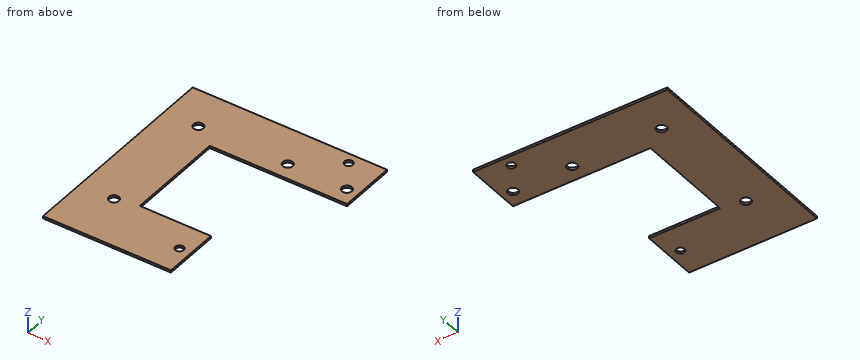
```python
from build123d import *

# Parameters (mm, degrees)
BASE_FLANGE1_DEPTH = 1
SKETCH3_R          = 2.1
SKETCH3_R_2        = 1.75
CUT_EXTRUDE1_DEPTH = 40
SKETCH4_R          = 1.75
CUT_EXTRUDE2_DEPTH = 10


# Sheet-metal steps are written as plain solids
with BuildPart() as part:
    # Sketch1 → Base-Flange1 (new body)
    with BuildSketch(Plane.XY):
        Polygon((0, 24), (-59, 24), (-59, -66), (-35, -66), (-5, -66), (-5, -42), (-35, -42), (-35, 0), (23, 0), (23, 24), align=None)
    extrude(amount=-BASE_FLANGE1_DEPTH)

    # Sketch3 → Cut-Extrude1 (cut)
    with BuildSketch(Plane.XY):
        with Locations((-44.600589414, -43.844308668)):
            Circle(SKETCH3_R)
        with Locations((-44.600589414, 6.892572586)):
            Circle(SKETCH3_R)
        with Locations((-6.896760866, 6.942572586)):
            Circle(SKETCH3_R)
        with Locations((18.060540453, 6.892572586)):
            Circle(SKETCH3_R)
        with Locations((10.002152137, 19.5)):
            Circle(SKETCH3_R_2)
    extrude(amount=-CUT_EXTRUDE1_DEPTH, mode=Mode.SUBTRACT)

    # Sketch4 → Cut-Extrude2 (cut)
    with BuildSketch(Plane.XY):
        with Locations((-9.791680506, -54)):
            Circle(SKETCH4_R)
    extrude(amount=-CUT_EXTRUDE2_DEPTH, mode=Mode.SUBTRACT)


solid = part.part
```
Geometry check sheet. Reference: the model listing, model coordinates, mm. Round coordinates to 2 decimals unless told otherwise and drop trailing zeros. Order: outer loops, then holes, each group sorted by start corner. A loop starts at its lowest first (then second) coordinate and runs counter-clockwise, first axis right, second up. Notation, with made-up numbers: (62.25, 16) -> (96.25, 16) arc R16 cw to (96.25, 38) -> close; hole circle Ø11 at (51, -40). An arc over 180 degrees is marked (long way). Return JSON: item names as keys, results as strings. Group by question number.
Q1. Section check A-A, the plane x = -20. Record the boundary of the cut face in (y, z).
Q2. Section check B-B, the plane y = -54. Record the boundary of the cut face in (x, z), plus the area to 3 significant figures.
Q3. Material ranges on probe 1 along Y at (x, z) = (-15, -0.55); probe 2 along X at (y, z) = (-44, -0.05); probe 3 along X at (y, z) = (7, -0.8), recorded low to high. Write a range as from..to.
Q4. Section check C-C, the plane z = -0.2. Record the boundary of the cut face in (x, y).
Q5. Section check D-D, the plane y = -17. Record the boundary of the cut face in (x, z).
Q6. Gauge pin test, flat end, axial feed: pin 1 (0.5 mm diameter, centred on y = -27.5, z = -0.5, fed in from +X). Record the tip position at first contact, or that the pin passes through.
Numbers:
{
 "1": {"outline": "(-66, -1) -> (-42, -1) -> (-42, 0) -> (-66, 0) -> close; (0, -1) -> (24, -1) -> (24, 0) -> (0, 0) -> close"},
 "2": {"outline": "(-59, -1) -> (-11.54, -1) -> (-11.54, 0) -> (-59, 0) -> close; (-8.04, -1) -> (-5, -1) -> (-5, 0) -> (-8.04, 0) -> close", "area": "50.5 mm^2"},
 "3": {"probe 1": "-66..-42, 0..24", "probe 2": "-59..-46.69, -42.51..-5", "probe 3": "-59..-46.7, -42.5..-9, -4.8..15.96, 20.16..23"},
 "4": {"outline": "(-59, -66) -> (-5, -66) -> (-5, -42) -> (-35, -42) -> (-35, 0) -> (23, 0) -> (23, 24) -> (-59, 24) -> close; hole circle Ø4.2 at (-44.6, -43.84); hole circle Ø4.2 at (-44.6, 6.89); hole circle Ø3.5 at (-9.79, -54); hole circle Ø4.2 at (-6.9, 6.94); hole circle Ø3.5 at (10, 19.5); hole circle Ø4.2 at (18.06, 6.89)"},
 "5": {"outline": "(-59, -1) -> (-35, -1) -> (-35, 0) -> (-59, 0) -> close"},
 "6": {"pin 1": "x = -35"}
}
